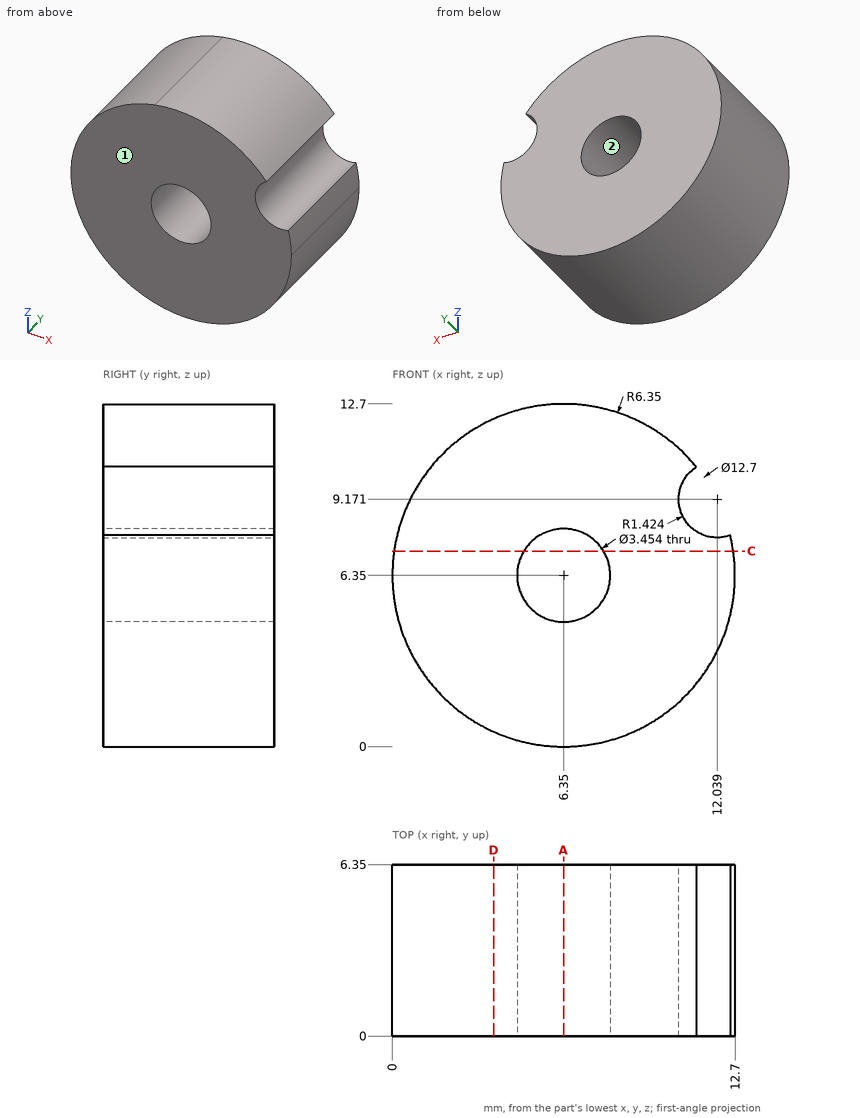
The drawing under review shows one solid part. Ordinate dimensions are in mm from its lowest x, y, z. Round coordinates to 2 decimals unless told otherwise and drop trailing zeros. Order: outer loops, then holes, each group sorted by start corner. A loop starts at its lowest first (then second) coordinate and runs counter-clockwise, first axis right, second up. Notation, with made-up numbers: (-7.75, 83) - (46.25, 83) arc R11 cw to (46.25, 100) - close; hole circle Ø2 at (30.5, 60.5). An arc over 180 degrees is marked (long way). Return JSON: item names as keys, results as strings.
Q1. Consider section C-C on z = 7.25. Write out the cut boundary in (x, y).
Computed values:
{"outline": "(0.06, 0) - (4.88, 0) - (4.88, 6.35) - (0.06, 6.35) - close; (7.82, 0) - (12.64, 0) - (12.64, 6.35) - (7.82, 6.35) - close"}
Q2. Wall thickness on L1, parallel to X at y = 2.75, z = 6.35; L2, parallel to X at y = 3.25, z = 7.25 (1 decimal): over which ranges is each line inside the solid? List them lowest first. Write a range as [from, to].
Computed values:
{"L1": "x = [0, 4.62], [8.08, 12.7]", "L2": "x = [0.1, 4.9], [7.8, 12.6]"}
Q3. The part is to be moulded in two halves that separate along Z. For the marked faces 1 and 2, say which applies: pulls with the +Z half, pulls with the -Z half, needs draft (parallel to the pull), parting line crosses it, or undercut.
Computed values:
{"face 1": "needs draft", "face 2": "undercut"}
Q4. Consider section D-D on x = 3.75. Write out the cut boundary in (y, z).
Computed values:
{"outline": "(0, 0.56) - (6.35, 0.56) - (6.35, 12.14) - (0, 12.14) - close"}
Q5. For pin 1 Ø3 at (y, z) = (4, 9) entering from -X (1 decimal), flat-tipped, find the tip position at first contact; note if it passes through.
Computed values:
{"pin 1": "stops at x = 0.1"}
Q6. Consider section A-A on x = 6.35. Write out the cut boundary in (y, z).
Computed values:
{"outline": "(0, 0) - (6.35, 0) - (6.35, 4.62) - (0, 4.62) - close; (0, 8.08) - (6.35, 8.08) - (6.35, 12.7) - (0, 12.7) - close"}
